from build123d import *

# Parameters (mm, degrees)
PAD_DEPTH       = 3
SKETCH001_W     = 10
SKETCH001_H     = 3
POCKET_DEPTH    = 3.001
SKETCH002_W     = 3
SKETCH002_H     = 10
POCKET001_DEPTH = 280.835483


with BuildPart() as part:
    # Sketch → Pad (new body)
    with BuildSketch(Plane.YZ):
        Polygon((-60.5, 0), (60.5, 0), (60.5, 10), (66.5, 10), (66.5, 40), (-66.5, 40), (-66.5, 10), (-60.5, 10), align=None)
    extrude(amount=PAD_DEPTH)

    # Sketch001 (on Face10 of Pad) → Pocket (cut, through all)
    with BuildSketch(Plane.YZ.offset(3)):
        with Locations((-51.5, 6.5)):
            Rectangle(SKETCH001_W, SKETCH001_H)
        with Locations((-31.5, 6.5)):
            Rectangle(SKETCH001_W, SKETCH001_H)
        with Locations((-11.5, 6.5)):
            Rectangle(SKETCH001_W, SKETCH001_H)
        with Locations((8.5, 6.5)):
            Rectangle(SKETCH001_W, SKETCH001_H)
        with Locations((28.5, 6.5)):
            Rectangle(SKETCH001_W, SKETCH001_H)
        with Locations((48.5, 6.5)):
            Rectangle(SKETCH001_W, SKETCH001_H)
    extrude(amount=-POCKET_DEPTH, mode=Mode.SUBTRACT)

    # Sketch002 (on Face5 of Pocket) → Pocket001 (cut, through all)
    with BuildSketch(Plane.YZ.offset(3)):
        with Locations((-62, 25)):
            Rectangle(SKETCH002_W, SKETCH002_H)
    pocket001 = extrude(amount=-POCKET001_DEPTH, mode=Mode.SUBTRACT)

    # Mirrored: Pocket001 across Sketch002 V_Axis
    add(pocket001.mirror(Plane(origin=(3, 0, 0), x_dir=(1, 0, 0), z_dir=(0, 1, 0))), mode=Mode.SUBTRACT)


solid = part.part
The listing builds one solid part. Answer for the finished solid, in the listing's coordinates (mm). A direction names the side the tool comes from. Round coordinates to 2 decimals unless told otherwise and drop trailing zeros. Write each loop counter-clockwise with the first axis right and the second up, starting at its lowest first coordinate (ties: lowest second). Pieces come first, ordered by that corner, then holes. Notation, with made-up numbers: (-37, 54.5) - (-27, 54.5) arc R31 cw to (-27, 82.5) - close; hole circle Ø4 at (53.5, 24.5). An arc over 180 degrees is marked (long way). Use a Markdown table: item, result. Add a question column.
1. The part is cut by section A-A (z = 28). Write down the section's boundary in (x, y), and give its area (3 significant figures).
2. The part is cut by section C-C (x = 1.1). Give the number of separate pieces and of enclosed holes in the cut face, and give its area (3 significant figures).
3. For a pull along Y with two mould halves and no side action, classify faces 4 (the face through (0, -1, 20)), 5 (the face through (2, -52, 5)) as +Y half, -Y half, draft (parallel to the pull), parting line (faces both ways), or undercut.
4. A tool of negligible diameter and unlimited length cuts with its end or side. For faces 1 (the face through (1, -64, 10)), 2 (the face through (2, 48, 5)), 3 (the face through (1, 1, 40)), from which of +Z, -Z, +X, -X, +Y, -Y can it reach the whole face along a straight path? Write none if from no direction.
5. Flat-ended cylindrical pins translate along their axes: P1, Ø1.5, axis at x = 1, z = 6, coming from the +Y side; P2, Ø1.5, axis at x = 2, z = 6, coming from the -Y side. Find the tip coordinate at first contact, or state that the pin passes through.
6. The part is cut by section B-B (y = 7.5). Write down the section's boundary in (x, z), and give its area (3 significant figures).
7. Consider line 1 (Y direction, x = 2.1, z = 24); line 2 (Z direction, x = 1.3, y = 48); line 3 (Z direction, x = 1.8, y = 61). Determine where each line is inside the solid, lowest interval first.
Reported:
| question | item | result |
|---|---|---|
| 1 | outline | (0, -66.5) - (3, -66.5) - (3, -63.5) - (0, -63.5) - close; (0, -60.5) - (3, -60.5) - (3, 60.5) - (0, 60.5) - close; (0, 63.5) - (3, 63.5) - (3, 66.5) - (0, 66.5) - close |
| 1 | area | 381 mm^2 |
| 2 | separate pieces | 1 |
| 2 | enclosed holes | 8 |
| 2 | area | 4,960 mm^2 |
| 3 | face 4 | draft |
| 3 | face 5 | undercut |
| 4 | face 1 | -Z, +X, -X, -Y |
| 4 | face 2 | +X, -X |
| 4 | face 3 | +Z, +X, -X, +Y, -Y |
| 5 | P1 | y = 60.5 |
| 5 | P2 | y = -60.5 |
| 6 | outline | (0, 0) - (3, 0) - (3, 5) - (0, 5) - close; (0, 8) - (3, 8) - (3, 40) - (0, 40) - close |
| 6 | area | 111 mm^2 |
| 7 | line 1 | -66.5 to -63.5, -60.5 to 60.5, 63.5 to 66.5 |
| 7 | line 2 | 0 to 5, 8 to 40 |
| 7 | line 3 | 10 to 20, 30 to 40 |
